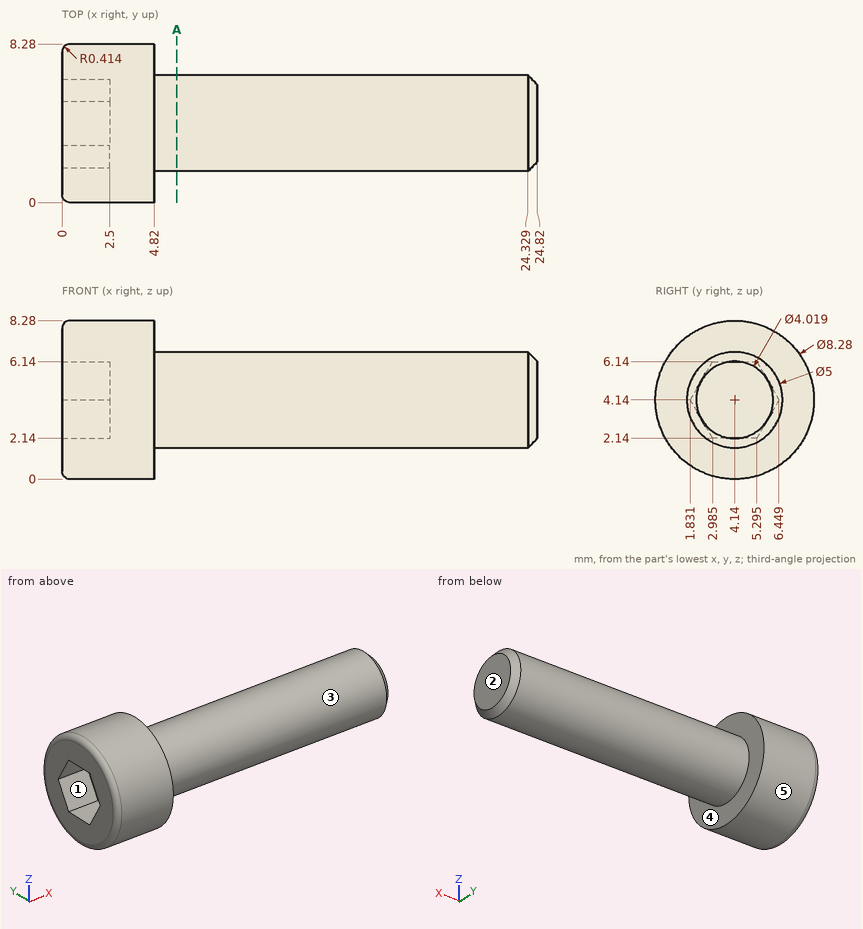
Geometry check sheet. Reference: drawing and pictorial views, mm from the part's lowest x, y, z. A direction names the side the tool comes from. Round coordinates to 2 decimals unless told otherwise and drop trailing zeros. Write each loop counter-clockwise with the first axis right and the second up, starting at its lowest first coordinate (ties: lowest second). Pieces come first, ordered by that corner, then holes. Notation, with made-up numbers: (29, 15) -> (59, 15) arc R19 cw to (59, 26) -> close; hole circle Ø8 at (-22, 66). An arc over 180 degrees is marked (long way). One line per question, with ' | ' between items. Start each with the question number.
1. Scan lines: line 1 along X through (y, z) = (2, 1.75); line 2 along X through (y, z) = (3.5, 6); line 3 along Y through (x, z) = (13.5, 4) (1 decimal). Record each from-to range of solid material in increasing order. Write a range as from..to.
2. Depth check by flat-ended pin: pin 1 (3 mm diameter, centred on x = 16.5, y = 6, fed in from +Z); pin 2 (1 mm diameter, centred on x = 8.5, z = 3.5, fed in from -Y); pin 3 (1.5 mm diameter, centred on x = 5, z = 2, fed in from -Y). Enter the tip coordinate at first touch or a pass-through.
3. Release check for a two-part mould opening along Z. For the marked faces 1, 2 and 3 record: +Z half, -Z half, draft (parallel to the pull), parting line (faces both ways), or undercut.
4. Set-up check for the marked faces 4 and 5: record each of +Z, -Z, +X, -X, +Y, -Y from which the full face is reachable in a straight line by a thin tool's end or side.
5. Sectioned sample at A-A, the plane x = 6. Record the cut outline in (y, z).
Taken from the geometry:
1) line 1: x = 0..4.82 | line 2: x = 2.5..24.82 | line 3: y = 1.6..6.6
2) pin 1: stops at z = 6.61 | pin 2: stops at y = 1.64 | pin 3: stops at y = 0.25
3) face 1: undercut | face 2: draft | face 3: parting line
4) face 4: +X | face 5: +X, -X
5) outline: circle Ø5 at (4.14, 4.14)
